from build123d import *

# Parameters (mm, degrees)
SKETCH1_W           = 203.2
SKETCH1_H           = 152.4
BOSS_EXTRUDE1_DEPTH = 76.2
SKETCH2_R           = 12.7
CUT_EXTRUDE1_DEPTH  = 25.4


with BuildPart() as part:
    # Sketch1 → Boss-Extrude1 (new body)
    with BuildSketch(Plane(origin=(0, 0, 0), x_dir=(1, 0, 0), z_dir=(0, 1, 0))):
        Rectangle(SKETCH1_W, SKETCH1_H)
    extrude(amount=BOSS_EXTRUDE1_DEPTH)

    # Sketch2 → Cut-Extrude1 (cut)
    with BuildSketch(Plane(origin=(0, 76.2, 0), x_dir=(1, 0, 0), z_dir=(0, 1, 0))):
        with Locations((-76.2, -50.8)):
            Circle(SKETCH2_R)
        with Locations((-76.2, 0)):
            Circle(SKETCH2_R)
        with Locations((-76.2, 50.8)):
            Circle(SKETCH2_R)
        with Locations((76.2, 50.8)):
            Circle(SKETCH2_R)
        with Locations((76.2, -50.8)):
            Circle(SKETCH2_R)
        with Locations((76.2, 0)):
            Circle(SKETCH2_R)
        with BuildLine():
            Line((-19.05, -38.1), (-19.05, 38.1))
            ThreePointArc((-19.05, 38.1), (0, 57.15), (19.05, 38.1))
            Line((19.05, 38.1), (19.05, -38.1))
            ThreePointArc((19.05, -38.1), (0, -57.15), (-19.05, -38.1))
        make_face()
    extrude(amount=-CUT_EXTRUDE1_DEPTH, mode=Mode.SUBTRACT)


solid = part.part
Work out the finished part from the listing and answer in its coordinate system (mm). A direction names the side the tool comes from. Round coordinates to 2 decimals unless told otherwise and drop trailing zeros. Loops run counter-clockwise (first coordinate to the right, second up) from the corner with the lowest first, then second, coordinate; pieces in that order, holes last. Notation, with made-up numbers: M 60.25,-36 L 74.25,-36 A17 cw 74.25,-22 Z; hole C 14.25,-12 d10. An arc over 180 degrees is marked long. One line per question, with ' | ' between items. Start each with the question number.
(1) A cutting plane is placed at B-B on z = 0. Write down the section's boundary in (x, y), plus the area to 3 significant figures.
(2) A cutting plane is placed at A-A on x = 76.2. Write down the section's boundary in (y, z), plus the area to 3 significant figures.
(3) Find the intervals of material crossed by line 1 (Z direction, x = 76, y = 64); line 2 (Z direction, x = 68.5, y = 63); line 3 (X direction, y = 60, z = -50), in increasing order.
(4) For a pull along X with two mould halves and no side action, classify faces 3 (the face through (21, 76.2, -1)), 4 (the face through (76, 50.8, 51)), 5 (the face through (-101.6, 38, 1)) as released by +X, released by -X, zero draft, split by the parting line, or undercut.
(5) A cutting plane is placed at C-C on x = 0. Write down the section's boundary in (y, z).
(6) A flat-ended cylindrical pin translates along its axis: pin 1 Ø15 at (x, z) = (76.2, 0) entering from +Y. Find the tip coordinate at first contact, or state that the pin passes through.
(7) A tool of negligible diameter and unlimited length cuts with its end or side. For faces 1 (the face through (-1, 0, -1)), 2 (the face through (0, 50.8, -1)), from which of +Z, -Z, +X, -X, +Y, -Y can it reach the whole face along a straight path? Write none if from no direction.
Geometry check:
1) outline: M -101.6,0 L 101.6,0 L 101.6,76.2 L 88.9,76.2 L 88.9,50.8 L 63.5,50.8 L 63.5,76.2 L 19.05,76.2 L 19.05,50.8 L -19.05,50.8 L -19.05,76.2 L -63.5,76.2 L -63.5,50.8 L -88.9,50.8 L -88.9,76.2 L -101.6,76.2 Z | area: 13,200 mm²
2) outline: M 0,-76.2 L 76.2,-76.2 L 76.2,-63.5 L 50.8,-63.5 L 50.8,-38.1 L 76.2,-38.1 L 76.2,-12.7 L 50.8,-12.7 L 50.8,12.7 L 76.2,12.7 L 76.2,38.1 L 50.8,38.1 L 50.8,63.5 L 76.2,63.5 L 76.2,76.2 L 0,76.2 Z | area: 9,680 mm²
3) line 1: z = -76.2 to -63.5, -38.1 to -12.7, 12.7 to 38.1, 63.5 to 76.2 | line 2: z = -76.2 to -60.9, -40.7 to -10.1, 10.1 to 40.7, 60.9 to 76.2 | line 3: x = -101.6 to -88.87, -63.53 to -14.88, 14.88 to 63.53, 88.87 to 101.6
4) face 3: zero draft | face 4: undercut | face 5: released by -X
5) outline: M 0,-76.2 L 76.2,-76.2 L 76.2,-57.15 L 50.8,-57.15 L 50.8,57.15 L 76.2,57.15 L 76.2,76.2 L 0,76.2 Z
6) pin 1: stops at y = 50.8
7) face 1: +Z, -Z, +X, -X, -Y | face 2: +Y
